Check sheet for the modelled part. Datum: model origin and axes. Units: mm. A direction names the side the tool comes from. Round coordinates to 2 decimals unless told otherwise and drop trailing zeros. Order: outer loops, then holes, each group sorted by start corner. A loop starts at its lowest first (then second) coordinate and runs counter-clockwise, first axis right, second up.
Q1. Cross-section at D-D on y = -16. Record the cut outline in (x, z).
Q2. Mould release check, pull along Y, two halves, no side actions. Record for faces 4 (the flat face through (38.1, -3.4, 0.3)), 5 (the cylindrical face through (19.317, 0.266, 12.837)), 6 (the cylindrical face through (19.317, -8.193, 2.314)): +Y half, -Y half, draft (parallel to the pull), parting line (faces both ways), or undercut.
Q3. Set-up check for faces 1 (the flat face through (19, 17, 0.794)), 2 (the flat face through (19, -17, 0.794)), 3 (the flat face through (0, -3.4, 0.3)): record each of +Z, -Z, +X, -X, +Y, -Y from which the full face is reachable in a straight line by a thin tool's end or side.
Q4. Cross-section at C-C on x = 18. Record the cut outline in (y, z) (3 decimals), then the cut area to 3 significant figures.
Q5. Scan lines: probe 1 along Y at (x, z) = (35.5, 6.5); probe 2 along Y at (x, z) = (5, 11.75); probe 3 along Z at (x, y) = (36, -19.5). Record each from-to range of solid material in increasing order.
Q6. Cross-section at B-B on y = -4. Record the cut outline in (x, z), then the cut area to 3 significant figures.
Q7. Cross-section at A-A on z = 8.75. Record the cut outline in (x, y).
Q8. Depth check by flat-ended pin: P1, Ø8.5, axis at x = 10.5, y = 18.5, coming from the +Z side; P2, Ø1, axis at x = 6.5, z = 5, coming from the +Y side; P3, Ø1, axis at x = 31.5, z = 10, coming from the +Y side. Enter the tip coordinate at first touch or a pass-through.
from build123d import *

# Parameters (mm, degrees)
F1_DEPTH = 38.1
F3_DEPTH = 38.101
F4_R     = 5.08
F5_DEPTH = 38.101


with BuildPart() as f1:
    # F0 (on Right) → F1 (new body)
    with BuildSketch(Plane.YZ):
        with BuildLine():
            Line((-22.225, 0.79375), (-22.225, 0))
            Line((-22.225, 0), (0, 0))
            Line((0, 0), (22.225, 0))
            Line((22.225, 0), (22.225, 0.79375))
            Line((22.225, 0.79375), (3.827324, 0.79375))
            ThreePointArc((3.827324, 0.79375), (0, 13.096875), (-3.827324, 0.79375))
            Line((-3.827324, 0.79375), (-22.225, 0.79375))
        make_face()
    extrude(amount=F1_DEPTH)

    # F2 (on face) → F3 (cut, through all)
    with BuildSketch(Plane.YZ.offset(38.1)):
        with BuildLine():
            Line((-1.354594, 0), (1.354594, 0))
            ThreePointArc((1.354594, 0), (0, 12.842875), (-1.354594, 0))
        make_face()
    extrude(amount=-F3_DEPTH, mode=Mode.SUBTRACT)

    # F4
    f4_edges = [f1.edges().sort_by_distance(p)[0] for p in [
        (19.05, -3.827324, 0.79375),
        (19.05, 3.827324, 0.79375),
    ]]
    fillet(f4_edges, radius=F4_R)

    # F2 (on face) → F5 (cut, through all)
    with BuildSketch(Plane.YZ.offset(38.1)):
        with BuildLine():
            Line((-1.354594, 0), (1.354594, 0))
            ThreePointArc((1.354594, 0), (0, 12.842875), (-1.354594, 0))
        make_face()
    extrude(amount=-F5_DEPTH, mode=Mode.SUBTRACT)


solid = f1.part
Results found:
1. outline: (0, 0) - (38.1, 0) - (38.1, 0.79) - (0, 0.79) - close
2. face 4: draft
2. face 5: undercut
2. face 6: -Y half
3. face 1: +Z, +X, -X, +Y
3. face 2: +Z, +X, -X, -Y
3. face 3: +Z, -Z, -X, +Y, -Y
4. outline: (-22.225, 0) - (-1.355, 0) arc R6.493 cw (long way) to (1.355, 0) - (22.225, 0) - (22.225, 0.794) - (11.817, 0.794) arc R5.08 cw to (6.741, 6.078) arc R6.747 ccw (long way) to (-6.741, 6.078) arc R5.08 cw to (-11.817, 0.794) - (-22.225, 0.794) - close
4. area: 60.6 mm2
5. probe 1: y = -6.75 to -6.49, 6.49 to 6.75
5. probe 2: y = -4.04 to -3.61, 3.61 to 4.04
5. probe 3: z = 0 to 0.79
6. outline: (0, 0) - (38.1, 0) - (38.1, 1.24) - (0, 1.24) - close; (0, 11.46) - (38.1, 11.46) - (38.1, 11.78) - (0, 11.78) - close
6. area: 59.2 mm2
7. outline: (0, -6.31) - (38.1, -6.31) - (38.1, -6.03) - (0, -6.03) - close; (0, 6.03) - (38.1, 6.03) - (38.1, 6.31) - (0, 6.31) - close
8. P1: stops at z = 0.79
8. P2: stops at y = 6.93
8. P3: stops at y = 5.97
